Part model, mm, in its own coordinate system. A direction names the side the tool comes from. Give positions to 0.01 mm unless a question says otherwise; leave off trailing zeros. Write each loop counter-clockwise with the first axis right and the second up, starting at its lowest first coordinate (ties: lowest second). Pieces come first, ordered by that corner, then holes. Notation, with made-up numbers: (-9.75, 11) - (21.25, 11) arc R33 cw to (21.25, 43) - close; hole circle Ø6 at (-10, -15.75). An arc over 180 degrees is marked (long way). Answer as a JSON object with one key per item and string values. Group by question number.
```python
from build123d import *

# Parameters (mm, degrees)
EXTRUDE_1_DEPTH               = 41.25
CUT_EXTRUDE_1_DEPTH           = 58.02151458
CUT_EXTRUDE_1_DEPTH_BACK      = 58.02151458
SKETCH_4_R                    = 1.75
CUT_EXTRUDE_2_DEPTH           = 10
HOLE_WIZARD_M31_REACH         = 75.336
HOLE_WIZARD_M31_BORE_R        = 1.25
HOLE_WIZARD_M32_D             = 2.5
SKETCH_10_R                   = 1.9
EXTRUDE_2_DEPTH               = 2.2
HOLE_WIZARD_M33_D             = 2.5
HOLE_WIZARD_M31_2_D           = 3.4
HOLE_WIZARD_M31_2_DEPTH       = 8.5
HOLE_WIZARD_M31_2_CSINK_D     = 6.3
HOLE_WIZARD_M31_2_CSINK_ANGLE = 90
HOLE_WIZARD_M31_2_TIP         = 1.021463052


with BuildPart() as part:
    # Эскиз1 → Бобышка-Вытянуть1 (new, symmetric)
    with BuildSketch(Plane.XY):
        with BuildLine():
            Line((-26.625, 29), (-26.625, 3))
            ThreePointArc((-26.625, 3), (-25.746320344, 0.878679656), (-23.625, 0))
            Line((-23.625, 0), (23.625, 0))
            ThreePointArc((23.625, 0), (25.746320344, 0.878679656), (26.625, 3))
            Line((26.625, 3), (26.625, 29))
            Line((26.625, 29), (24.125, 29))
            Line((24.125, 29), (24.125, 2.5))
            Line((24.125, 2.5), (-24.125, 2.5))
            Line((-24.125, 2.5), (-24.125, 29))
            Line((-24.125, 29), (-26.625, 29))
        make_face()
    extrude(amount=EXTRUDE_1_DEPTH, both=True)

    # Эскиз3 → Вырез-Вытянуть1 (cut, two sides: drawn at the far end of the back side and taken through both)
    with BuildSketch(Plane(origin=(0, 0, 0), x_dir=(0, 0, -1), z_dir=(1, 0, 0)).offset(-CUT_EXTRUDE_1_DEPTH_BACK)):
        Polygon((41.25, 21), (41.25, 29), (33.5, 29), align=None)
        Polygon((-41.25, 21), (-41.25, 29), (-33.5, 29), align=None)
    extrude(amount=CUT_EXTRUDE_1_DEPTH + CUT_EXTRUDE_1_DEPTH_BACK, mode=Mode.SUBTRACT)

    # Эскиз4 → Вырез-Вытянуть2 (cut)
    with BuildSketch(Plane.XZ):
        with Locations((-19.5, -37.6)):
            Circle(SKETCH_4_R)
        with Locations((-19.5, 37.6)):
            Circle(SKETCH_4_R)
        with Locations((19.5, 37.6)):
            Circle(SKETCH_4_R)
        with Locations((19.5, -37.6)):
            Circle(SKETCH_4_R)
    extrude(amount=-CUT_EXTRUDE_2_DEPTH, mode=Mode.SUBTRACT)

    # Hole Wizard M31 bore → Hole Wizard M31 (cut, up to next)
    with BuildSketch(Plane(origin=(26.625, 0, 0), x_dir=(0, 0, -1), z_dir=(1, 0, 0)), mode=Mode.PRIVATE) as hole_wizard_m31_sk1:
        with Locations((37.75, 18)):
            Circle(HOLE_WIZARD_M31_BORE_R)
    hole_wizard_m31_tool1 = extrude(hole_wizard_m31_sk1.sketch, amount=-HOLE_WIZARD_M31_REACH, mode=Mode.PRIVATE) & part.part
    # Hole Wizard M31 bore → Hole Wizard M31 (cut, up to next)
    with BuildSketch(Plane(origin=(26.625, 0, 0), x_dir=(0, 0, -1), z_dir=(1, 0, 0)), mode=Mode.PRIVATE) as hole_wizard_m31_sk2:
        with Locations((-37.75, 18)):
            Circle(HOLE_WIZARD_M31_BORE_R)
    hole_wizard_m31_tool2 = extrude(hole_wizard_m31_sk2.sketch, amount=-HOLE_WIZARD_M31_REACH, mode=Mode.PRIVATE) & part.part
    add(hole_wizard_m31_tool1.solids().sort_by_distance((26.625, 18, -37.75))[0], mode=Mode.SUBTRACT)
    add(hole_wizard_m31_tool2.solids().sort_by_distance((26.625, 18, 37.75))[0], mode=Mode.SUBTRACT)

    # Отверстие обработанное метчиком M32 (through all)
    with Locations(Plane.ZY.offset(26.625)):
        with Locations((-37.75, 18), (37.75, 18)):
            Hole(HOLE_WIZARD_M32_D / 2)

    # Эскиз10 → Бобышка-Вытянуть2 (add)
    with BuildSketch(Plane(origin=(0, 2.5, 0), x_dir=(1, 0, 0), z_dir=(0, 1, 0))):
        with Locations(Location((19.5, 31, 0), (0, 0, 90))):
            Circle(SKETCH_10_R)
        with Locations(Location((19.5, -31, 0), (0, 0, 90))):
            Circle(SKETCH_10_R)
        with Locations(Location((-19.5, -31, 0), (0, 0, 90))):
            Circle(SKETCH_10_R)
        with Locations(Location((-19.5, 31, 0), (0, 0, 90))):
            Circle(SKETCH_10_R)
    extrude(amount=EXTRUDE_2_DEPTH)

    # Отверстие обработанное метчиком M33 (through all)
    with Locations(Plane(origin=(0, 4.7, 0), x_dir=(1, 0, 0), z_dir=(0, 1, 0))):
        with Locations((19.5, 31), (-19.5, 31), (19.5, -31), (-19.5, -31)):
            Hole(HOLE_WIZARD_M33_D / 2)

    # Hole Wizard M31 2
    with Locations(Plane(origin=(26.625, 0, 0), x_dir=(0, 0, -1), z_dir=(1, 0, 0))):
        with Locations((-8, 14)):
            CounterSinkHole(HOLE_WIZARD_M31_2_D / 2, HOLE_WIZARD_M31_2_CSINK_D / 2, depth=HOLE_WIZARD_M31_2_DEPTH, counter_sink_angle=HOLE_WIZARD_M31_2_CSINK_ANGLE)
            with Locations((0, 0, -(HOLE_WIZARD_M31_2_DEPTH + HOLE_WIZARD_M31_2_TIP / 2))):  # 118° drill point
                Cone(0, HOLE_WIZARD_M31_2_D / 2, HOLE_WIZARD_M31_2_TIP, mode=Mode.SUBTRACT)


solid = part.part
```
1) Saw through at A-A (y = 14). List the corners of the cut face in (x, z) (3 decimals).
2) Drop flat-ended pins along their axis: P1, Ø24, axis at x = 10.5, z = -12, coming from the +Y side; P2, Ø1.1, axis at x = 18.5, z = -31, coming from the +Y side; P3, Ø2, axis at x = -19.5, z = -37.6, coming from the +Y side. Give the stop position or say it passes through.
3) Saw through at D-D (y = 24.5). List the corners of the cut face in (x, z) (3 decimals), and give its area (3 significant figures).
4) Saw through at B-B (x = -19.5). List the corners of the cut face in (y, z), and give its area (3 significant figures).
5) Which spindle directions (+Z, -Z, +X, -X, +Y, -Y) get a long thin tool onto all of the face, cutting with end or side? Do faces 1 (the flat face through (-25, 29, 0)), 2 (the flat face through (21, 4.7, 31)). Say none if no direction does.
6) Drill centre lines: line 1 along X through (y, z) = (2.9, 31) (3 decimals); line 2 along Z through (x, y) = (-19.5, 2.25); line 3 along X through (y, z) = (23.5, 31.5) (3 decimals). Where is each one in solid material? Low to high. Write a range as from..to.
7) Saw through at C-C (z = 8). List the corners of the cut face in (x, y) (3 decimals).
8) Two-plate mould, pull along Z, no slides. Class faces 3 (the flat face through (-25.392, 25.056, -37.321)), 4 (the flat face through (-18, 4.7, 31)), 5 (the cylindrical face through (18.929, 3.585, 29.188)): +Z half, -Z half, draft (parallel to the pull), parting line (faces both ways), or undercut.
Checks:
{
 "1": {"outline": "(-26.625, -41.25) - (-24.125, -41.25) - (-24.125, 41.25) - (-26.625, 41.25) - close; (24.125, -41.25) - (26.625, -41.25) - (26.625, 4.85) - (25.175, 6.3) - (24.125, 6.3) - close; (24.125, 9.7) - (25.175, 9.7) - (26.625, 11.15) - (26.625, 41.25) - (24.125, 41.25) - close"},
 "2": {"P1": "y = 2.5", "P2": "y = 4.7", "P3": "through"},
 "3": {"outline": "(-26.625, -37.859) - (-24.125, -37.859) - (-24.125, 37.859) - (-26.625, 37.859) - close; (24.125, -37.859) - (26.625, -37.859) - (26.625, 37.859) - (24.125, 37.859) - close", "area": "379 mm2"},
 "4": {"outline": "(0, -41.25) - (2.5, -41.25) - (2.5, -39.35) - (0, -39.35) - close; (0, -35.85) - (2.5, -35.85) - (2.5, -32.9) - (4.7, -32.9) - (4.7, -32.25) - (0, -32.25) - close; (0, -29.75) - (4.7, -29.75) - (4.7, -29.1) - (2.5, -29.1) - (2.5, 29.1) - (4.7, 29.1) - (4.7, 29.75) - (0, 29.75) - close; (0, 32.25) - (4.7, 32.25) - (4.7, 32.9) - (2.5, 32.9) - (2.5, 35.85) - (0, 35.85) - close; (0, 39.35) - (2.5, 39.35) - (2.5, 41.25) - (0, 41.25) - close", "area": "182 mm2"},
 "5": {"face 1": "+Z, -Z, +X, -X, +Y", "face 2": "+Z, -Z, +Y"},
 "6": {"line 1": "-26.623..-24.125, -21.4..-20.75, -18.25..-17.6, 17.6..18.25, 20.75..21.4, 24.125..26.623", "line 2": "-41.25..-39.35, -35.85..-32.25, -29.75..29.75, 32.25..35.85, 39.35..41.25", "line 3": "-26.625..-24.125, 24.125..26.625"},
 "7": {"outline": "(-26.625, 3) arc R3 ccw to (-23.625, 0) - (23.625, 0) arc R3 ccw to (26.625, 3) - (26.625, 10.85) - (25.175, 12.3) - (24.125, 12.3) - (24.125, 2.5) - (-24.125, 2.5) - (-24.125, 29) - (-26.625, 29) - close; (24.125, 15.7) - (25.175, 15.7) - (26.625, 17.15) - (26.625, 29) - (24.125, 29) - close"},
 "8": {"face 3": "-Z half", "face 4": "draft", "face 5": "undercut"}
}
